Source: CAD feature listing. Evaluate the final solid. Frame: model axes, mm. Coordinates: 2 decimals unless noted, no trailing zeros. Write each loop counter-clockwise with the first axis right and the second up, starting at its lowest first coordinate (ties: lowest second). Pieces come first, ordered by that corner, then holes. Notation, with made-up numbers: M 53,21 L 64,21 A10 cw 64,31 Z; hole C 28.5,-31 d2. An arc over 180 degrees is marked long. Write item = value, one per line. Start each with the question number.
1. Section query A-A (y = 3). Output: boundary loops of the cut face in (x, z).
2. Section query B-B (x = 8.5). Output: boundary loops of the cut face in (y, z), then the cut area to 3 significant figures.
3. Section query C-C (y = 34.5). Output: boundary loops of the cut face in (x, z), then the cut area to 3 significant figures.
4. Line query: line 1 along Y through (x, z) = (13.5, 0.9); line 2 along Y through (x, z) = (8.5, 1.85); line 3 along Y through (x, z) = (9.25, 2.25). Output: solid intervals per line, ascending.
5. Section query D-D (z = 1.2). Output: boundary loops of the cut face in (x, y).
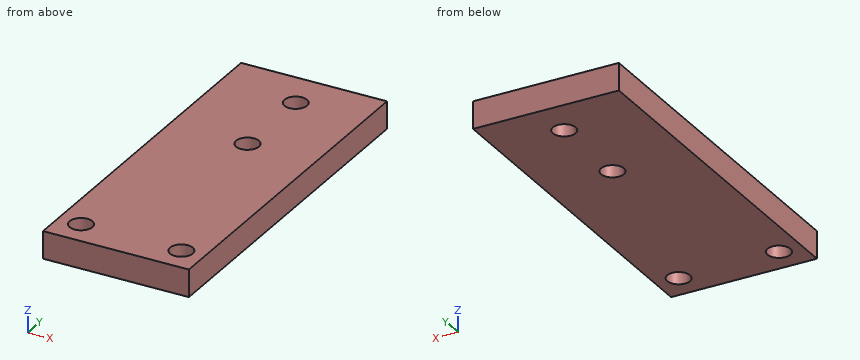
Autodesk Inventor part; units mm, degrees
ref_plane "YZ Plane" through (0, 0, 0) normal (1, 0, 0) x (0, 1, 0)
ref_plane "XZ Plane" through (0, 0, 0) normal (0, 1, 0) x (-1, 0, 0)
ref_plane "XY Plane" through (0, 0, 0) normal (0, 0, 1) x (1, 0, 0)
sketch "Sketch1" plane through (0, 0, 0) normal (0, 0, 1) x (1, 0, 0)
  line L0 (0, 0) -> (16, 0)
  line L1 (16, 0) -> (16, 39)
  line L2 (16, 39) -> (0, 39)
  line L3 (0, 39) -> (0, 0)
  line L4 (8, 32.7385) -> (8, -1.6019) construction
  line L5 (8, 0) -> (8, 3) construction
  line L6 (8, 3) -> (-6.2893, 3) construction
  line L7 (-6.2893, 3) -> (30.6517, 3) construction
  line L8 (8, 3) -> (13.5, 3) construction
  line L9 (13.5, 3) -> (13.5, 7.8913) construction
  line L10 (13.5, 7.8913) -> (2.5, 7.8913) construction
  line L11 (2.5, 7.8913) -> (2.5, 1.5) construction
  circle A0 centre (2.5, 3) radius 1.25
  circle A1 centre (13.5, 3) radius 1.25
  line L12 (8, 0) -> (8, 25) construction
  line L13 (8, 25) -> (38.3893, 25) construction
  line L14 (38.3893, 25) -> (38.3893, 34.5) construction
  line L15 (38.3893, 34.5) -> (16, 34.5) construction
  line L16 (16, 34.5) -> (8.5, 34.5) construction
  line L17 (8.5, 34.5) -> (8.5, 22.056) construction
  circle A2 centre (8.5, 34.5) radius 1.25
  circle A3 centre (8.5, 25) radius 1.25
  dimension "d0" = 16
  dimension "d1" = 39
  dimension "d2" = 3
  dimension "d3" = 5.5
  dimension "d4" = 11
  dimension "d5" = 2.5
  dimension "d6" = 2.5
  dimension "d7" = 25
  dimension "d8" = 9.5
  dimension "d9" = 7.5
  dimension "d10" = 2.5
  dimension "d11" = 2.5
extrude "Extrusion1" add sketch "Sketch1" along normal blind 3
properties part number "bart x endstop bracket plain switch v1"
Results are:
q1.outline = M 0,0 L 1.25,0 L 1.25,3 L 0,3 Z; M 3.75,0 L 12.25,0 L 12.25,3 L 3.75,3 Z; M 14.75,0 L 16,0 L 16,3 L 14.75,3 Z
q2.outline = M 0,0 L 23.75,0 L 23.75,3 L 0,3 Z; M 26.25,0 L 33.25,0 L 33.25,3 L 26.25,3 Z; M 35.75,0 L 39,0 L 39,3 L 35.75,3 Z
q2.area = 102 mm^2
q3.outline = M 0,0 L 7.25,0 L 7.25,3 L 0,3 Z; M 9.75,0 L 16,0 L 16,3 L 9.75,3 Z
q3.area = 40.5 mm^2
q4.line_1 = 0 to 1.75, 4.25 to 39
q4.line_2 = 0 to 23.75, 26.25 to 33.25, 35.75 to 39
q4.line_3 = 0 to 24, 26 to 33.5, 35.5 to 39
q5.outline = M 0,0 L 16,0 L 16,39 L 0,39 Z; hole C 2.5,3 d2.5; hole C 8.5,25 d2.5; hole C 8.5,34.5 d2.5; hole C 13.5,3 d2.5
